Here's how the part is built. I have some questions about the finished solid (model axes, mm). Round coordinates to 2 decimals unless told otherwise and drop trailing zeros. Order: outer loops, then holes, each group sorted by start corner. A loop starts at its lowest first (then second) coordinate and runs counter-clockwise, first axis right, second up. Notation, with made-up numbers: (18.5, -35) -> (37.5, -35) arc R21 cw to (37.5, -17) -> close; hole circle Ø9 at (32, 12.25). An arc over 180 degrees is marked (long way). One line per item, written item: value.
```python
from build123d import *

# Parameters (mm, degrees)
THREADSCHEMATIC_START     = -4.953
THREADSCHEMATIC_OUTLINE_R = 3.2639
THREADSCHEMATIC_DEPTH     = 4.953


# Read off the part's stored shape, not the designer's step: ThreadSchematic
with BuildPart() as part:
    # ThreadSchematic outline → ThreadSchematic (new body)
    with BuildSketch(Plane.XY.offset(THREADSCHEMATIC_START)):
        Polygon((6.35, 3.666174209), (0, 7.332348419), (-6.35, 3.666174209), (-6.35, -3.666174209), (0, -7.332348419), (6.35, -3.666174209), align=None)
        Circle(THREADSCHEMATIC_OUTLINE_R, mode=Mode.SUBTRACT)
    extrude(amount=THREADSCHEMATIC_DEPTH)

    # Sketch3 → Double-Chamfer (revolve, cut)
    with BuildSketch(Plane(origin=(0, 0, 0), x_dir=(0, 0, -1), z_dir=(1, 0, 0))):
        Polygon((4.953, 6.35), (4.15925, 7.332348419), (4.15925, 20.032348419), (17.653, 20.032348419), (17.653, 6.35), align=None)
        Polygon((0.79375, 20.032348419), (-12.7, 20.032348419), (-12.7, 6.35), (0, 6.35), (0.79375, 7.332348419), align=None)
    revolve(axis=Axis((0, 0, 0), (0, 0, -1)), mode=Mode.SUBTRACT)

    # EndChamferSke → EndChamfer (revolve, cut)
    with BuildSketch(Plane(origin=(0, 0, 0), x_dir=(0, 0, -1), z_dir=(1, 0, 0)), mode=Mode.PRIVATE) as endchamfer_sk:
        Polygon((4.9276, 3.96875), (4.384704588, 3.193415), (4.9784, 3.193415), (4.9784, 3.96875), align=None)
        Polygon((-0.0508, 3.96875), (0, 3.96875), (0.542895412, 3.193415), (-0.0508, 3.193415), align=None)
    revolve(endchamfer_sk.sketch.rotate(Axis((0, 0, -25.037505729), (0, 0, -1)), 90), axis=Axis((0, 0, -25.037505729), (0, 0, -1)), mode=Mode.SUBTRACT)


solid = part.part
```
Q1. I need wall thicknesses on line 1 along X through (y, z) = (0.5, -4.5); line 2 along Y through (x, z) = (-0.75, -3.8); line 3 along X through (y, z) = (-2.25, -0.95). Which ranges of each line are inside material? Lowest first, please.
Answers:
line 1: -6.35 to -3.32, 3.32 to 6.35
line 2: -6.9 to -3.18, 3.18 to 6.9
line 3: -6.35 to -2.36, 2.36 to 6.35
Q2. I want a section at A-A on z = -2.75. Write out the boundary of the cut face in (x, y), then the cut area to 3 significant figures.
Answers:
outline: (-6.35, -3.67) -> (0, -7.33) -> (6.35, -3.67) -> (6.35, 3.67) -> (0, 7.33) -> (-6.35, 3.67) -> close; hole circle Ø6.53 at (0, 0)
area: 106 mm2
Q3. If we mould it in two halves opening along Y, with no side actions, what happens to faces 1 (the face through (-0.708, -3.186, -2.491)), 2 (the face through (-3.219, -5.474, -2.511)), 3 (the face through (-3.131, 5.525, -2.511))? For each: pulls with the +Y half, pulls with the -Y half, needs draft (parallel to the pull), parting line crosses it, or undercut.
Answers:
face 1: undercut
face 2: pulls with the -Y half
face 3: pulls with the +Y half
Q4. For P1, Ø5, axis at x = 0, y = 0, coming from the +Z side; P2, Ø1.5, axis at x = 2, z = -1, coming from the +Y side, each with a flat end and sliding along its axis, tell me the tip position at first contact or that it passes through.
Answers:
P1: through
P2: y = 6.61
